Model file for the job. Use its own axes, mm. Coordinates: 2 decimals unless noted, no trailing zeros. Loops run counter-clockwise (first coordinate to the right, second up) from the corner with the lowest first, then second, coordinate; pieces in that order, holes last.
Autodesk Fusion 360 part; units mm, degrees
sketch "Sketch1" plane through (0, 0, 0) normal (1, 0, 0) x (0, 1, 0)
  circle A0 centre (0, 0) radius 0.5
  line L0 (0.325, -0.325) -> (-0.325, -0.325)
  line L1 (-0.325, -0.325) -> (-0.325, 0.325)
  line L2 (-0.325, 0.325) -> (0.325, 0.325)
  line L3 (0.325, 0.325) -> (0.325, -0.325)
  line L4 (0.325, -0.325) -> (-0.325, 0.325) construction
  line L5 (-0.325, -0.325) -> (0.325, 0.325) construction
  dimension "d1" = 1
  dimension "d2" = 0.65
  dimension "d3" = 0.65
extrude "Extrude1" add sketch "Sketch1" along normal blind 13 contours A0 | L0 L1 L2 L3
sketch "Sketch2" plane through (13, 0, 0) normal (1, 0, 0) x (0, 1, 0)
  circle A0 centre (0, 0) radius 0.5
  line L0 (0.325, -0.325) -> (-0.325, -0.325)
  line L1 (-0.325, -0.325) -> (-0.325, 0.325)
  line L2 (-0.325, 0.325) -> (0.325, 0.325)
  line L3 (0.325, 0.325) -> (0.325, -0.325)
  line L4 (0.325, -0.325) -> (-0.325, 0.325) construction
  line L5 (-0.325, -0.325) -> (0.325, 0.325) construction
  dimension "d8" = 0.65
  dimension "d9" = 0.65
extrude "Extrude2" add sketch "Sketch2" along normal blind 1.445 contours L0 L1 L2 L3
extrude "Extrude3" add sketch "Sketch1" against normal blind 1.445 contours L0 L1 L2 L3
sketch "Sketch3" plane through (0, 0, -0.325) normal (0, 0, -1) x (1, 0, 0)
  line L0 (13, 0.325) -> (13, -0.325)
  line L1 (13, -0.325) -> (14.445, -0.325)
  line L2 (14.445, -0.325) -> (14.445, 0.325)
  line L3 (14.445, 0.325) -> (13, 0.325)
  line L4 (14.445, 0.325) -> (13.795, 0.325)
  line L5 (13.795, 0.325) -> (13.795, -0.325)
  line L6 (13.795, -0.325) -> (14.445, -0.325)
  line L7 (14.445, -0.325) -> (14.445, 0.325)
  line L8 (14.445, 0.325) -> (13.795, -0.325) construction
  line L9 (13.795, 0.325) -> (14.445, -0.325) construction
  point P0 (14.12, 0)
  dimension "d14" = 0.65
  dimension "d15" = 0.65
sketch "Sketch4" plane through (0, 0, -0.325) normal (0, 0, -1) x (1, 0, 0)
  line L0 (0, -0.325) -> (0, 0.325)
  line L1 (0, 0.325) -> (-1.445, 0.325)
  line L2 (-1.445, 0.325) -> (-1.445, -0.325)
  line L3 (-1.445, -0.325) -> (0, -0.325)
  line L4 (-0.795, -0.325) -> (-1.445, -0.325)
  line L5 (-1.445, -0.325) -> (-1.445, 0.325)
  line L6 (-1.445, 0.325) -> (-0.795, 0.325)
  line L7 (-0.795, 0.325) -> (-0.795, -0.325)
  line L8 (-0.795, -0.325) -> (-1.445, 0.325) construction
  line L9 (-1.445, -0.325) -> (-0.795, 0.325) construction
  point P0 (-1.12, 0)
  dimension "d17" = 0.65
  dimension "d18" = 0.65
extrude "Extrude4" add sketch "Sketch4" sketch "Sketch3" along normal blind 2.75 contours L1 L2 L3 L4 L5 L6 L7 of sketch 2 contours L1 L2 L3 L4 L5 L6 L7
fillet "Fillet1" radius 0.5 2 edges at (-0.795, 0, -0.325) (13.795, 0, -0.325)
fillet "Fillet2" radius 1 2 edges at (-1.445, 0, 0.325) (14.445, 0, 0.325)
fillet "Fillet3" radius 0.2 28 edges at (-1.12, -0.325, -3.075) (-0.795, 0, -3.075) (-1.12, 0.325, -3.075) (-1.445, 0, -3.075) (-0.6486, -0.325, -0.4714) (-0.795, -0.325, -1.95) (-0.2225, -0.325, 0.325) (-1.1521, -0.325, 0.0321) (-1.445, -0.325, -1.875) (-0.2225, 0.325, 0.325) (-1.1521, 0.325, 0.0321) (-1.445, 0.325, -1.875) (-0.6486, 0.325, -0.4714) (-0.795, 0.325, -1.95) (13.2225, -0.325, 0.325) (14.1521, -0.325, 0.0321) (14.445, -0.325, -1.875) (13.795, -0.325, -1.95) (13.6486, -0.325, -0.4714) (14.445, 0.325, -1.875) (14.1521, 0.325, 0.0321) (13.2225, 0.325, 0.325) (13.6486, 0.325, -0.4714) (13.795, 0.325, -1.95) (14.12, 0.325, -3.075) (14.445, 0, -3.075) (14.12, -0.325, -3.075) (13.795, 0, -3.075)
equation "d1 = width"
equation "d2 = d3"
equation "d3 = d1 * 0.65"
equation "width = 1 mm"
equation "baseLenght = 13 mm"
equation "d6 = baseLenght"
equation "d8 = width * 0.65"
equation "d9 = d8"
equation "d14 = width * 0.65"
equation "d15 = d14"
equation "d17 = width * 0.65"
equation "d18 = d17"
equation "d26 = 0.2 * width"
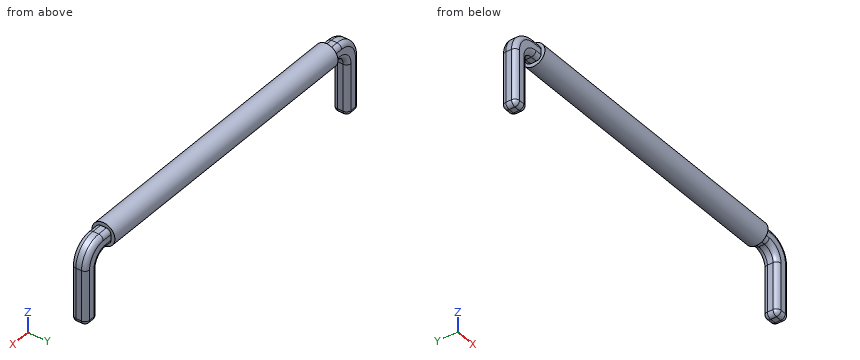
Q1. Slice it at B-B (x = 5.5). List the corners of the cut face in (y, z).
Answers:
outline: circle Ø1 at (0, 0)
Q2. Flat gauge pins, fed straight in: P1, Ø1, axis at x = -1, z = -1, coming from the +Y side (3 decimals); P2, Ø1, axis at x = 13.5, z = -1, coming from the -Y side (3 decimals); P3, Ø0.5, axis at y = 0, z = 0, coming from the -X side. Where does each tip first touch, or does it go through?
Answers:
P1: stops at y = 0.325
P2: stops at y = -0.325
P3: stops at x = -1.35
Q3. Drill centre lines: line 1 (X direction, y = 0, z = -1) (3 decimals); line 2 (Z direction, x = 6.5, y = 0.05); line 3 (Z direction, x = 4.25, y = -0.25). Where is each one in solid material? Low to high.
Answers:
line 1: x = -1.445 to -0.795, 13.795 to 14.445
line 2: z = -0.5 to 0.5
line 3: z = -0.43 to 0.43
Q4. Slice it at A-A (z = -2.7). List the corners of the cut face in (x, y) (3 decimals).
Answers:
outline: (-1.445, -0.125) arc R0.2 ccw to (-1.245, -0.325) - (-0.995, -0.325) arc R0.2 ccw to (-0.795, -0.125) - (-0.795, 0.125) arc R0.2 ccw to (-0.995, 0.325) - (-1.245, 0.325) arc R0.2 ccw to (-1.445, 0.125) - close; (13.795, -0.125) arc R0.2 ccw to (13.995, -0.325) - (14.245, -0.325) arc R0.2 ccw to (14.445, -0.125) - (14.445, 0.125) arc R0.2 ccw to (14.245, 0.325) - (13.995, 0.325) arc R0.2 ccw to (13.795, 0.125) - close
